```python
from build123d import *

# Parameters (mm, degrees)
SKETCH_1_R             = 80
EXTRUDE_1_DEPTH        = 2
SKETCH_2_R             = 1.6
CUT_EXTRUDE_445_DEPTH  = 2
SKETCH_3_R             = 1.35
SKETCH_3_W             = 56
SKETCH_3_H             = 15
SKETCH_3_W_2           = 15
SKETCH_3_H_2           = 58
CUT_EXTRUDE_949_DEPTH  = 2
SKETCH_4_R             = 1.6
CUT_EXTRUDE_1375_DEPTH = 2
SKETCH_5_R             = 1.1
CUT_EXTRUDE_1819_DEPTH = 2
FILLET_2_R             = 3


with BuildPart() as part:
    # 草图1 → 凸台-拉伸1 (new body)
    with BuildSketch(Plane(origin=(0, 0, 0), x_dir=(1, 0, 0), z_dir=(0, 1, 0))):
        Circle(SKETCH_1_R)
    extrude(amount=EXTRUDE_1_DEPTH)

    # 草图2 → Cut-Extrude 445 (cut)
    with BuildSketch(Plane(origin=(0, 2, 0), x_dir=(1, 0, 0), z_dir=(0, 1, 0))):
        with Locations((-62.5, 35)):
            Circle(SKETCH_2_R)
        with Locations((-62.5, -35)):
            Circle(SKETCH_2_R)
        with Locations((62.5, -35)):
            Circle(SKETCH_2_R)
        with Locations((62.5, 35)):
            Circle(SKETCH_2_R)
    extrude(amount=-CUT_EXTRUDE_445_DEPTH, mode=Mode.SUBTRACT)

    # 草图3 → Cut-Extrude 949 (cut)
    with BuildSketch(Plane(origin=(0, 2, 0), x_dir=(1, 0, 0), z_dir=(0, 1, 0))):
        with Locations((-24.5, 19)):
            Circle(SKETCH_3_R)
        with Locations((-24.5, -39)):
            Circle(SKETCH_3_R)
        with Locations((24.5, -39)):
            Circle(SKETCH_3_R)
        with Locations((24.5, 19)):
            Circle(SKETCH_3_R)
        with Locations((0, 60)):
            Rectangle(SKETCH_3_W, SKETCH_3_H)
        with Locations((46, -10)):
            Rectangle(SKETCH_3_W_2, SKETCH_3_H_2)
    extrude(amount=-CUT_EXTRUDE_949_DEPTH, mode=Mode.SUBTRACT)

    # 草图4 → Cut-Extrude 1375 (cut)
    with BuildSketch(Plane(origin=(0, 2, 0), x_dir=(1, 0, 0), z_dir=(0, 1, 0))):
        with Locations((-18, 35.65)):
            Circle(SKETCH_4_R)
        with Locations((0, 35.65)):
            Circle(SKETCH_4_R)
        with Locations((18, 35.65)):
            Circle(SKETCH_4_R)
        with Locations((18, -35.65)):
            Circle(SKETCH_4_R)
        with Locations((0, -35.65)):
            Circle(SKETCH_4_R)
        with Locations((-18, -35.65)):
            Circle(SKETCH_4_R)
    extrude(amount=-CUT_EXTRUDE_1375_DEPTH, mode=Mode.SUBTRACT)

    # 草图5 → Cut-Extrude 1819 (cut)
    with BuildSketch(Plane(origin=(0, 2, 0), x_dir=(1, 0, 0), z_dir=(0, 1, 0))):
        with Locations((-7, 9.25)):
            Circle(SKETCH_5_R)
        with Locations((7, 9.25)):
            Circle(SKETCH_5_R)
        with Locations((7, -9.25)):
            Circle(SKETCH_5_R)
        with Locations((-7, -9.25)):
            Circle(SKETCH_5_R)
    extrude(amount=-CUT_EXTRUDE_1819_DEPTH, mode=Mode.SUBTRACT)

    # 圆角2
    fillet_2_edges = [part.edges().sort_by_distance(p)[0] for p in [
        (38.5, 1, 39),
        (38.5, 1, -19),
        (53.5, 1, -19),
        (53.5, 1, 39),
        (-28, 1, -52.5),
        (-28, 1, -67.5),
        (28, 1, -67.5),
        (28, 1, -52.5),
    ]]
    fillet(fillet_2_edges, radius=FILLET_2_R)


solid = part.part
```
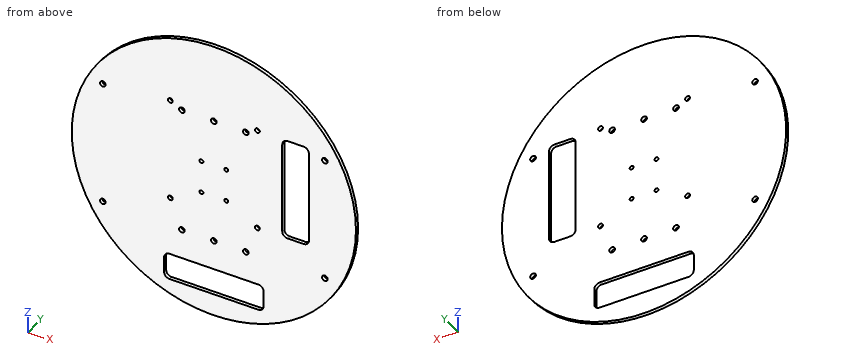
Can you work these out from the model? Positions are in its coordinate system, mm. Round coordinates to 2 decimals unless told otherwise and drop trailing zeros. Loops run counter-clockwise (first coordinate to the right, second up) from the corner with the lowest first, then second, coordinate; pieces in that order, holes last. Notation, with made-up numbers: (-32.75, 55.5) -> (-9.75, 55.5) arc R37 ccw to (-9.75, 91.5) -> close; hole circle Ø11 at (-9.75, 59.25). An arc over 180 degrees is marked (long way). Answer in a Markdown table with one row per item.
Item 1: Suppose I cut it at C-C, the plane x = 30. List the corners of the cut face in (y, z) for me.
Answer block:
| item | result |
|---|---|
| outline | (0, -74.16) -> (2, -74.16) -> (2, 74.16) -> (0, 74.16) -> close |
Item 2: Suppose I cut it at B-B, the plane y = 1.5. Give the number of separate pieces and of enclosed holes in the cut face, plus the area to 3 significant figures.
Answer block:
| item | result |
|---|---|
| separate pieces | 1 |
| enclosed holes | 20 |
| area | 18,300 mm² |
Item 3: Suppose I cut it at A-A, the plane z = -13.5. List the corners of the cut face in (x, y) for me.
Answer block:
| item | result |
|---|---|
| outline | (-78.85, 0) -> (38.5, 0) -> (38.5, 2) -> (-78.85, 2) -> close; (53.5, 0) -> (78.85, 0) -> (78.85, 2) -> (53.5, 2) -> close |
Item 4: Will these pins go through, and if not, where does the flat tip stop? P1, Ø1, axis at y = 1, z = 17, coming from the +X side; P2, Ø1, axis at y = 0.5, z = -1, coming from the -X side; P3, Ø1.9, axis at x = -18, z = -35.65, coming from the -Y side; P4, Ø1, axis at y = 0.5, z = -59.5, coming from the -X side.
Answer block:
| item | result |
|---|---|
| P1 | x = 78.28 |
| P2 | x = -80 |
| P3 | through |
| P4 | x = -54.03 |
Item 5: If I drill on probe 1 along Z at (x, y) = (7, 1.1); probe 2 along X at (y, z) = (1.15, -35); probe 3 along Z at (x, y) = (6, 0.45), over which ranges is the centre line in solid material (lowest first)?
Answer block:
| item | result |
|---|---|
| probe 1 | -79.69 to -67.5, -52.5 to -10.35, -8.15 to 8.15, 10.35 to 79.69 |
| probe 2 | -71.94 to -64.1, -60.9 to -19.46, -16.54 to -1.46, 1.46 to 16.54, 19.46 to 60.9, 64.1 to 71.94 |
| probe 3 | -79.77 to -67.5, -52.5 to -9.71, -8.79 to 8.79, 9.71 to 79.77 |
Item 6: Suppose I cut it at D-D, the plane z = 62. List the corners of the cut face in (x, y) for me.
Answer block:
| item | result |
|---|---|
| outline | (-50.56, 0) -> (50.56, 0) -> (50.56, 2) -> (-50.56, 2) -> close |
